from build123d import *

# Parameters (mm, degrees)
SKETCH1_W           = 40
SKETCH1_H           = 40
SKETCH1_R           = 1.5
BOSS_EXTRUDE1_DEPTH = 50
SKETCH1_3_W         = 15
SKETCH1_3_H         = 40
SKETCH1_3_R         = 1.5
BOSS_EXTRUDE2_DEPTH = 3
FILLET1_R           = 10
FILLET2_R           = 15


with BuildPart() as part:
    # Sketch1 → Boss-Extrude1 (new body)
    with BuildSketch(Plane(origin=(0, 0, 0), x_dir=(1, 0, 0), z_dir=(0, 1, 0))):
        Rectangle(SKETCH1_W, SKETCH1_H)
        with Locations(Location((-11.691342951, -6.75, 0), (0, 0, 270))):
            Circle(SKETCH1_R, mode=Mode.SUBTRACT)
        with Locations(Location((11.691342951, -6.75, 0), (0, 0, 270))):
            Circle(SKETCH1_R, mode=Mode.SUBTRACT)
        with Locations(Location((0, 13.5, 0), (0, 0, 270))):
            Circle(SKETCH1_R, mode=Mode.SUBTRACT)
    extrude(amount=BOSS_EXTRUDE1_DEPTH)

    # Sketch1<3> → Boss-Extrude2 (add)
    # profile 1 of 2: a face of its own
    with BuildSketch(Plane(origin=(0, 0, 0), x_dir=(1, 0, 0), z_dir=(0, 1, 0))):
        with Locations((-27.5, 0)):
            Rectangle(SKETCH1_3_W, SKETCH1_3_H)
        with Locations(Location((-25, -15, 0), (0, 0, 270))):
            Circle(SKETCH1_3_R, mode=Mode.SUBTRACT)
        with Locations(Location((-25, 15, 0), (0, 0, 270))):
            Circle(SKETCH1_3_R, mode=Mode.SUBTRACT)
    # profile 2 of 2: a face of its own
    with BuildSketch(Plane(origin=(0, 0, 0), x_dir=(1, 0, 0), z_dir=(0, 1, 0))):
        with Locations((27.5, 0)):
            Rectangle(SKETCH1_3_W, SKETCH1_3_H)
        with Locations(Location((25, -15, 0), (0, 0, 270))):
            Circle(SKETCH1_3_R, mode=Mode.SUBTRACT)
        with Locations(Location((25, 15, 0), (0, 0, 270))):
            Circle(SKETCH1_3_R, mode=Mode.SUBTRACT)
    extrude(amount=BOSS_EXTRUDE2_DEPTH)

    # Fillet1
    # the kernel refuses this fillet: 10 mm, written as the material it takes off along each edge
    with BuildSketch(Plane(origin=(35, 3, 37.853571071), x_dir=(0, -1, 0), z_dir=(0, 0, -1))) as fillet1_piece_1:
        with BuildLine():
            CenterArc((10, 7.141428429), FILLET1_R, 180, 45.572995999)
            Line((0, 7.141428429), (-0.2, 7.141428429))
            Line((-0.2, 7.141428429), (-0.2, 0))
            Line((-0.2, 0), (0, -0.2))
            ThreePointArc((0, -0.2), (1.5, -0.2), (2.86, -0.142828569))
            Line((2.86, -0.142828569), (3, 0))
        make_face()
    extrude(amount=75.707142143, mode=Mode.SUBTRACT)
    with BuildSketch(Plane(origin=(-35, 3, -37.853571071), x_dir=(1, 0, 0), z_dir=(0, 0, 1))) as fillet1_piece_2:
        with BuildLine():
            CenterArc((7.141428429, -10), FILLET1_R, 90, 45.572995999)
            Line((0, -3), (-0.142828569, -2.86))
            ThreePointArc((-0.142828569, -2.86), (-0.2, -1.5), (-0.2, 0))
            Line((-0.2, 0), (0, 0.2))
            Line((0, 0.2), (7.141428429, 0.2))
            Line((7.141428429, 0.2), (7.141428429, 0))
        make_face()
    extrude(amount=75.707142143, mode=Mode.SUBTRACT)

    # Fillet2
    fillet2_edges = [part.edges().sort_by_distance(p)[0] for p in [
        (-20, 26.5, -20),
        (20, 26.5, -20),
        (20, 26.5, 20),
        (-20, 26.5, 20),
    ]]
    fillet(fillet2_edges, radius=FILLET2_R)


solid = part.part
Could you check a few things on this model? Use its own coordinates, in mm. A direction names the side the tool comes from. Give positions to 0.01 mm unless a question says otherwise; leave off trailing zeros. Order: outer loops, then holes, each group sorted by start corner. A loop starts at its lowest first (then second) coordinate and runs counter-clockwise, first axis right, second up.
1. Suppose I cut it at B-B (x = 0). List the corners of the cut face in (y, z) for me, plus the area to 3 significant figures.
2. For faces 1 (the flat face through (-20, 26, 0)), 2 (the flat face through (0, 17, 20)), 3 (the cylindrical face through (15.49, 26.83, -15.72)), 4 (the cylindrical face through (15.49, 26.83, 15.72)), which set-ups out of +Z, -Z, +X, -X, +Y, -Y let a thin tool reach every point of the face, with its end or its side?
3. Suppose I cut it at D-D (y = 37). List the corners of the cut face in (x, z) for me.
4. I need wall thicknesses on L1, parallel to X at y = 12.5, z = 5.5; L2, parallel to X at y = 28, z = 6.75; L3, parallel to X at y = 35.5, z = 3. Which ranges of each line are inside material? Lowest first, please.
5. We'd pull the mould along X, two halves only. Please class faces 5 (the cylindrical face through (26.01, 1.48, 13.89)), 6 (the flat face through (20, 26, 0)), 7 (the flat face through (0, 50, 0)): pulls with the +X half, pulls with the -X half, needs draft (parallel to the pull), parting line crosses it, or undercut.
6. Suppose I cut it at A-A (x = 25). List the corners of the cut face in (y, z) for me, plus the area to 3 significant figures.
7. Suppose I cut it at C-C (z = 6.75). List the corners of the cut face in (x, y) for me, plus the area to 3 significant figures.
8. Will these pins go through, and if not, where does the flat tip stop? P1, Ø12, axis at x = -27, z = -5.5, coming from the +Y side; P2, Ø2, axis at x = -16, y = 9, coming from the -Z side; P3, Ø8, axis at y = 20, z = -1, coming from the +X side; P4, Ø4, axis at x = 11.69, z = 6.75, coming from the +Y side.
Solved:
1. outline: (0, -20) - (50, -20) - (50, -15) - (0, -15) - close; (0, -12) - (50, -12) - (50, 20) - (0, 20) - close
1. area: 1,850 mm2
2. face 1: +Z, -Z, -X, +Y
2. face 2: +Z, +X, -X, +Y, -Y
2. face 3: -Z, +X, +Y
2. face 4: +Z, +X, +Y
3. outline: (-20, -5) arc R15 ccw to (-5, -20) - (5, -20) arc R15 ccw to (20, -5) - (20, 5) arc R15 ccw to (5, 20) - (-5, 20) arc R15 ccw to (-20, 5) - close; hole circle Ø3 at (-11.69, 6.75); hole circle Ø3 at (0, -13.5); hole circle Ø3 at (11.69, 6.75)
4. L1: x = -19.99 to -12.52, -10.86 to 10.86, 12.52 to 19.99
4. L2: x = -19.9 to -13.19, -10.19 to 10.19, 13.19 to 19.9
4. L3: x = -20 to 20
5. face 5: undercut
5. face 6: pulls with the +X half
5. face 7: needs draft
6. outline: (0, -20) - (3, -20) - (3, -16.5) - (0, -16.5) - close; (0, -13.5) - (3, -13.5) - (3, 13.5) - (0, 13.5) - close; (0, 16.5) - (3, 16.5) - (3, 20) - (0, 20) - close
6. area: 102 mm2
7. outline: (-35, 0) - (-13.19, 0) - (-13.19, 50) - (-19.9, 50) - (-19.9, 3) - (-27.86, 3) arc R10 ccw to start; (-10.19, 0) - (10.19, 0) - (10.19, 50) - (-10.19, 50) - close; (13.19, 0) - (35, 0) arc R10 ccw to (27.86, 3) - (19.9, 3) - (19.9, 50) - (13.19, 50) - close
7. area: 1,770 mm2
8. P1: stops at y = 3
8. P2: stops at z = -16.18
8. P3: stops at x = 20
8. P4: stops at y = 50
